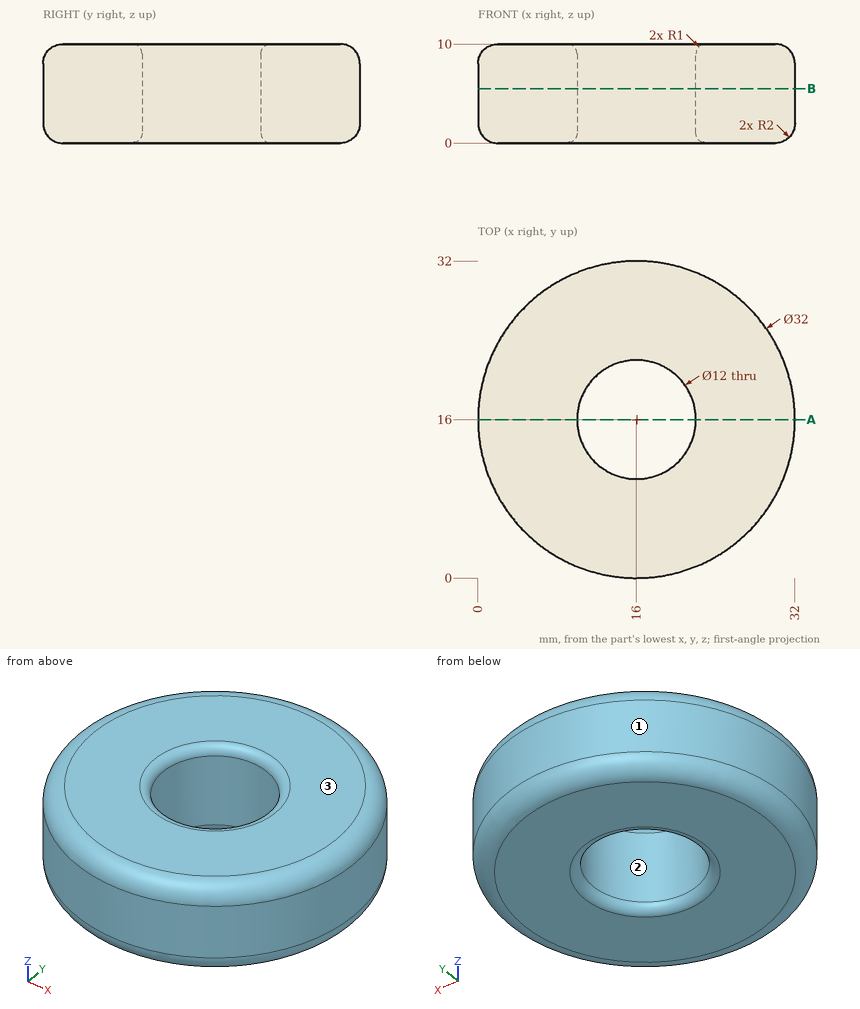
Part print with two shaded views. Sizes in mm from the minimum x, y, z corner. Round coordinates to 2 decimals unless told otherwise and drop trailing zeros. Loops run counter-clockwise (first coordinate to the right, second up) from the corner with the lowest first, then second, coordinate; pieces in that order, holes last. Notation, with made-up numbers: M -5.5,-29.5 L 10.5,-29.5 A23 ccw 10.5,3.5 Z; hole C 9.25,-16 d5. An arc over 180 degrees is marked long. Return JSON: item names as keys, results as strings. Group by question number.
(1) Mould opens along X. For the marked faces 1, 2 and 3 say: +X half, -X half, draft (parallel to the pull), parting line (faces both ways), or undercut.
(2) Saw through at B-B, the plane z = 5.5. List the corners of the cut face in (x, y).
(3) Saw through at A-A, the plane y = 16. List the corners of the cut face in (x, z).
(4) Drop flat-ended pins along their axis: P1, Ø2, axis at x = 27.5, z = 5.5, coming from the -Y side; P2, Ø1, axis at x = 22, z = 3, coming from the +Y side (3 decimals); P3, Ø1, axis at x = 27, y = 26, coming from the +Z side; P4, Ø12, axis at x = 26, y = 13.5, coming from the -Z side. Give the stop position or say it passes through.
(5) Wall check: probe 1 along Y at (x, z) = (16, 7.5); probe 2 along X at (y, z) = (21, 3.5); probe 3 along X at (y, z) = (18, 0.75). Give the ranges that are in metal, low to high. Write a range as [from, to].
Answer list:
{
 "1": {"face 1": "parting line", "face 2": "undercut", "face 3": "draft"},
 "2": {"outline": "C 16,16 d32; hole C 16,16 d12"},
 "3": {"outline": "M 0,2 A2 ccw 2,0 L 9,0 A1 ccw 10,1 L 10,9 A1 ccw 9,10 L 2,10 A2 ccw 0,8 Z; M 22,1 A1 ccw 23,0 L 30,0 A2 ccw 32,2 L 32,8 A2 ccw 30,10 L 23,10 A1 ccw 22,9 Z"},
 "4": {"P1": "y = 3.93", "P2": "y = 31.025", "P3": "z = 9.97", "P4": "z = 0"},
 "5": {"probe 1": "[0, 10], [22, 32]", "probe 2": "[0.8, 12.68], [19.32, 31.2]", "probe 3": "[0.57, 10.31], [21.69, 31.43]"}
}
